Could you check a few things on this drawing? It's one solid part, dimensions in mm from its lowest x, y, z. Coordinates: 2 decimals unless noted, no trailing zeros. Order: outer loops, then holes, each group sorted by start corner. A loop starts at its lowest first (then second) coordinate and runs counter-clockwise, first axis right, second up.
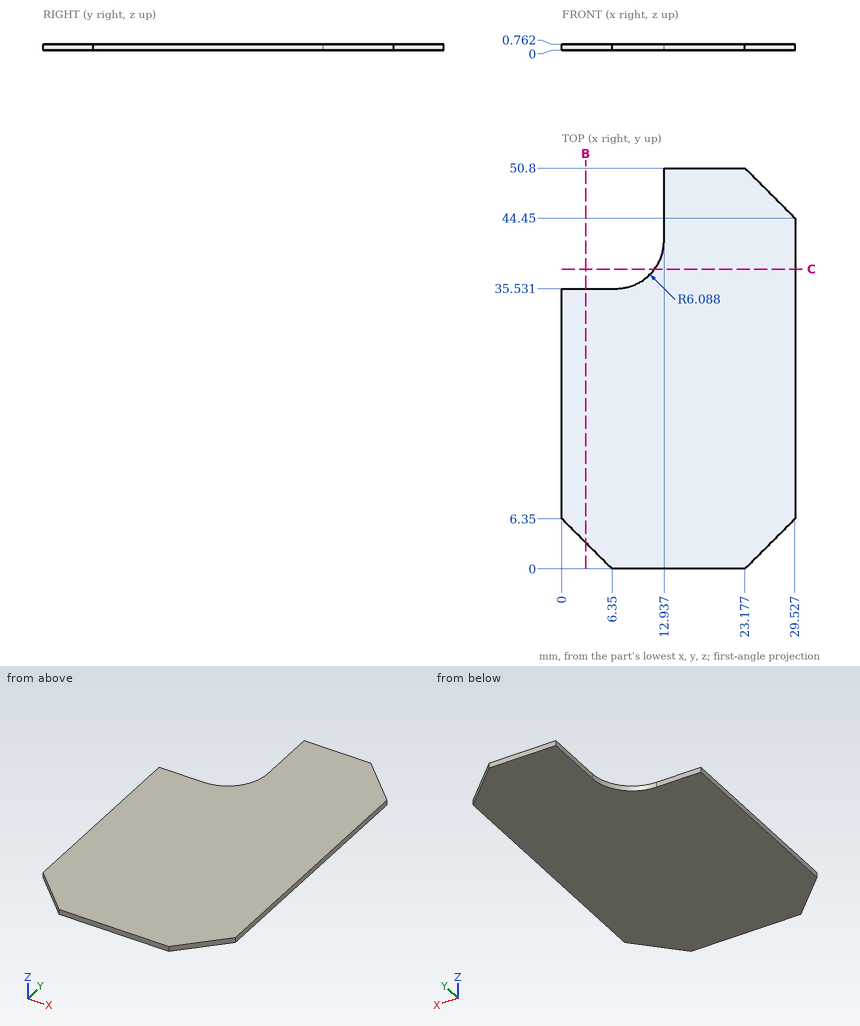
Item 1: I need wall thicknesses on line 1 (X direction, y = 43.5, z = 0.4); line 2 (Y direction, x = 8.75, z = 0.15) (1 decimal); line 3 (X direction, y = 36.5, z = 0.3) (1 decimal). Which ranges of each line are inside material? Lowest first, please.
Item 2: Suppose I cut it at C-C (y = 38). List the corners of the cut face in (x, z) for me (1 decimal).
Item 3: Suppose I cut it at B-B (x = 3). List the corners of the cut face in (y, z) for me.
Geometry results:
1. line 1: x = 12.94 to 29.53
1. line 2: y = 0 to 35.8
1. line 3: x = 10.1 to 29.5
2. outline: (11.7, 0) - (29.5, 0) - (29.5, 0.8) - (11.7, 0.8) - close
3. outline: (3.35, 0) - (35.53, 0) - (35.53, 0.76) - (3.35, 0.76) - close
